For this review, take the finished solid that the model builds, in its own axes (mm). Give positions to 0.01 mm unless a question says otherwise; leave off trailing zeros. Write each loop counter-clockwise with the first axis right and the second up, starting at its lowest first coordinate (ties: lowest second). Pieces come first, ordered by that corner, then holes. Notation, with made-up numbers: M 78.5,-1.5 L 90.5,-1.5 A7 ccw 90.5,10.5 Z; hole C -13.5,62.5 d8. An arc over 180 degrees is marked long. One line per item, written item: value. Start each with the question number.
Item 1: Consider section A-A, the plane y = 38.5. Write out the cut boundary in (x, z).
Item 2: To check wall thickness, follow probe 1 along Y at (x, z) = (0, 6.25); probe 2 along X at (y, z) = (-6.5, 8.25); probe 3 along Y at (x, z) = (-4, 4.5). State the ranges of each line that lie inside material, in increasing order.
Item 3: Consider section B-B, the plane z = 7.75. Give the number of separate pieces and of enclosed holes in the cut face, and give its area (3 significant figures).
Item 4: Consider section C-C, the plane y = -20. Write out the cut boundary in (x, z), and give its area (3 significant figures).
Item 5: Consider section D-D, the plane y = -37. Write out the cut boundary in (x, z), and give its area (3 significant figures).
Item 6: Clearance check with flat-ended pins moving along their axes: pin 1 Ø4 at (y, z) = (-26.5, 4.5) entering from -X; pin 2 Ø2 at (y, z) = (-18.5, 7.5) entering from -X; pin 3 Ø6.5 at (x, z) = (19, 6) entering from -Y. State where each tip first meets the part, or that it passes through.
Item 7: Mouldability with a two-part tool opening along X and no side actions: class faces 1 (the face through (9.82, -24.54, 6.26)), 2 (the face through (42.95, 8.66, 6.26)), 3 (the face through (0, -10, 0)), 4 (the face through (42.397, 13.352, 6.261)) as released by +X, released by -X, zero draft, split by the parting line, or undercut.
```python
from build123d import *

# Parameters (mm, degrees)
F0_R     = 44.45
F0_R_2   = 8.89
F1_DEPTH = 12.7


with BuildPart() as f1:
    # F0 (on Top) → F1 (new body)
    with BuildSketch(Plane.XY):
        Circle(F0_R)
        with BuildLine():
            Line((-30.756564, -31.205577), (-6.506943, -6.955956))
            ThreePointArc((-6.506943, -6.955956), (-5.291806, -7.919748), (-3.936366, -8.67356))
            Line((-3.936366, -8.67356), (-17.060166, -40.357217))
            ThreePointArc((-17.060166, -40.357217), (-24.34231, -36.430841), (-30.756564, -31.205577))
        make_face(mode=Mode.SUBTRACT)
        with BuildLine():
            Line((-16.473503, -40.600221), (-3.349702, -8.916564))
            ThreePointArc((-3.349702, -8.916564), (-1.858235, -9.34198), (-0.3175, -9.519707))
            Line((-0.3175, -9.519707), (-0.3175, -43.81385))
            ThreePointArc((-0.3175, -43.81385), (-8.547882, -42.973107), (-16.473503, -40.600221))
        make_face(mode=Mode.SUBTRACT)
        with BuildLine():
            Line((-40.357217, -17.060166), (-8.67356, -3.936366))
            ThreePointArc((-8.67356, -3.936366), (-7.919748, -5.291806), (-6.955956, -6.506943))
            Line((-6.955956, -6.506943), (-31.205577, -30.756564))
            ThreePointArc((-31.205577, -30.756564), (-36.430841, -24.34231), (-40.357217, -17.060166))
        make_face(mode=Mode.SUBTRACT)
        with BuildLine():
            ThreePointArc((-40.600221, -16.473503), (-42.973107, -8.547882), (-43.81385, -0.3175))
            Line((-43.81385, -0.3175), (-9.519707, -0.3175))
            ThreePointArc((-9.519707, -0.3175), (-9.34198, -1.858235), (-8.916564, -3.349702))
            Line((-8.916564, -3.349702), (-40.600221, -16.473503))
        make_face(mode=Mode.SUBTRACT)
        with BuildLine():
            ThreePointArc((0.3175, -9.519707), (1.858235, -9.34198), (3.349702, -8.916564))
            Line((3.349702, -8.916564), (16.473503, -40.600221))
            ThreePointArc((16.473503, -40.600221), (8.547882, -42.973107), (0.3175, -43.81385))
            Line((0.3175, -43.81385), (0.3175, -9.519707))
        make_face(mode=Mode.SUBTRACT)
        with BuildLine():
            ThreePointArc((3.936366, -8.67356), (5.291806, -7.919748), (6.506943, -6.955956))
            Line((6.506943, -6.955956), (30.756564, -31.205577))
            ThreePointArc((30.756564, -31.205577), (24.34231, -36.430841), (17.060166, -40.357217))
            Line((17.060166, -40.357217), (3.936366, -8.67356))
        make_face(mode=Mode.SUBTRACT)
        with BuildLine():
            ThreePointArc((6.955956, -6.506943), (7.919748, -5.291806), (8.67356, -3.936366))
            Line((8.67356, -3.936366), (40.357217, -17.060166))
            ThreePointArc((40.357217, -17.060166), (36.430841, -24.34231), (31.205577, -30.756564))
            Line((31.205577, -30.756564), (6.955956, -6.506943))
        make_face(mode=Mode.SUBTRACT)
        with BuildLine():
            ThreePointArc((8.916564, -3.349702), (9.34198, -1.858235), (9.519707, -0.3175))
            Line((9.519707, -0.3175), (43.81385, -0.3175))
            ThreePointArc((43.81385, -0.3175), (42.973107, -8.547882), (40.600221, -16.473503))
            Line((40.600221, -16.473503), (8.916564, -3.349702))
        make_face(mode=Mode.SUBTRACT)
        with BuildLine():
            Line((-40.600221, 16.473503), (-8.916564, 3.349702))
            ThreePointArc((-8.916564, 3.349702), (-9.34198, 1.858235), (-9.519707, 0.3175))
            Line((-9.519707, 0.3175), (-43.81385, 0.3175))
            ThreePointArc((-43.81385, 0.3175), (-42.973107, 8.547882), (-40.600221, 16.473503))
        make_face(mode=Mode.SUBTRACT)
        with BuildLine():
            Line((-31.205577, 30.756564), (-6.955956, 6.506943))
            ThreePointArc((-6.955956, 6.506943), (-7.919748, 5.291806), (-8.67356, 3.936366))
            Line((-8.67356, 3.936366), (-40.357217, 17.060166))
            ThreePointArc((-40.357217, 17.060166), (-36.430841, 24.34231), (-31.205577, 30.756564))
        make_face(mode=Mode.SUBTRACT)
        with BuildLine():
            Line((-17.060166, 40.357217), (-3.936366, 8.67356))
            ThreePointArc((-3.936366, 8.67356), (-5.291806, 7.919748), (-6.506943, 6.955956))
            Line((-6.506943, 6.955956), (-30.756564, 31.205577))
            ThreePointArc((-30.756564, 31.205577), (-24.34231, 36.430841), (-17.060166, 40.357217))
        make_face(mode=Mode.SUBTRACT)
        with BuildLine():
            ThreePointArc((-16.473503, 40.600221), (-8.547882, 42.973107), (-0.3175, 43.81385))
            Line((-0.3175, 43.81385), (-0.3175, 9.519707))
            ThreePointArc((-0.3175, 9.519707), (-1.858235, 9.34198), (-3.349702, 8.916564))
            Line((-3.349702, 8.916564), (-16.473503, 40.600221))
        make_face(mode=Mode.SUBTRACT)
        Circle(F0_R_2, mode=Mode.SUBTRACT)
        with BuildLine():
            Line((43.81385, 0.3175), (9.519707, 0.3175))
            ThreePointArc((9.519707, 0.3175), (9.34198, 1.858235), (8.916564, 3.349702))
            Line((8.916564, 3.349702), (40.600221, 16.473503))
            ThreePointArc((40.600221, 16.473503), (42.973107, 8.547882), (43.81385, 0.3175))
        make_face(mode=Mode.SUBTRACT)
        with BuildLine():
            Line((40.357217, 17.060166), (8.67356, 3.936366))
            ThreePointArc((8.67356, 3.936366), (7.919748, 5.291806), (6.955956, 6.506943))
            Line((6.955956, 6.506943), (31.205577, 30.756564))
            ThreePointArc((31.205577, 30.756564), (36.430841, 24.34231), (40.357217, 17.060166))
        make_face(mode=Mode.SUBTRACT)
        with BuildLine():
            Line((16.473503, 40.600221), (3.349702, 8.916564))
            ThreePointArc((3.349702, 8.916564), (1.858235, 9.34198), (0.3175, 9.519707))
            Line((0.3175, 9.519707), (0.3175, 43.81385))
            ThreePointArc((0.3175, 43.81385), (8.547882, 42.973107), (16.473503, 40.600221))
        make_face(mode=Mode.SUBTRACT)
        with BuildLine():
            Line((30.756564, 31.205577), (6.506943, 6.955956))
            ThreePointArc((6.506943, 6.955956), (5.291806, 7.919748), (3.936366, 8.67356))
            Line((3.936366, 8.67356), (17.060166, 40.357217))
            ThreePointArc((17.060166, 40.357217), (24.34231, 36.430841), (30.756564, 31.205577))
        make_face(mode=Mode.SUBTRACT)
    extrude(amount=F1_DEPTH)


solid = f1.part
```
Model answer:
1. outline: M -22.22,0 L -20.92,0 L -20.92,12.7 L -22.22,12.7 Z; M -16.29,0 L -15.6,0 L -15.6,12.7 L -16.29,12.7 Z; M -0.32,0 L 0.32,0 L 0.32,12.7 L -0.32,12.7 Z; M 15.6,0 L 16.29,0 L 16.29,12.7 L 15.6,12.7 Z; M 20.92,0 L 22.22,0 L 22.22,12.7 L 20.92,12.7 Z
2. probe 1: y = -44.45 to -8.89, 8.89 to 44.45
2. probe 2: x = -43.97 to -43.33, -16.52 to -14.86, -6.96 to -6.06, 6.06 to 6.96, 14.86 to 16.52, 43.33 to 43.97
2. probe 3: y = -44.27 to -43.63, -10.49 to -8.83, -8.64 to -7.94, 7.94 to 8.64, 8.83 to 10.49, 43.63 to 44.27
3. separate pieces: 1
3. enclosed holes: 17
3. area: 561 mm2
4. outline: M -39.7,0 L -38.98,0 L -38.98,12.7 L -39.7,12.7 Z; M -20.45,0 L -19.55,0 L -19.55,12.7 L -20.45,12.7 Z; M -8.63,0 L -7.94,0 L -7.94,12.7 L -8.63,12.7 Z; M -0.32,0 L 0.32,0 L 0.32,12.7 L -0.32,12.7 Z; M 7.94,0 L 8.63,0 L 8.63,12.7 L 7.94,12.7 Z; M 19.55,0 L 20.45,0 L 20.45,12.7 L 19.55,12.7 Z; M 38.98,0 L 39.7,0 L 39.7,12.7 L 38.98,12.7 Z
4. area: 66.4 mm2
5. outline: M -24.63,0 L -23.47,0 L -23.47,12.7 L -24.63,12.7 Z; M -15.67,0 L -14.98,0 L -14.98,12.7 L -15.67,12.7 Z; M -0.32,0 L 0.32,0 L 0.32,12.7 L -0.32,12.7 Z; M 14.98,0 L 15.67,0 L 15.67,12.7 L 14.98,12.7 Z; M 23.47,0 L 24.63,0 L 24.63,12.7 L 23.47,12.7 Z
5. area: 55.1 mm2
6. pin 1: stops at x = -37.09
6. pin 2: stops at x = -40.86
6. pin 3: stops at y = -41.57
7. face 1: undercut
7. face 2: undercut
7. face 3: zero draft
7. face 4: split by the parting line
